from build123d import *

# Parameters (mm, degrees)
PAD_DEPTH    = 3
POCKET_DEPTH = 5
CHAMFER_SIZE = 1
FILLET_R     = 1


with BuildPart() as part:
    # Sketch → Pad (new body)
    with BuildSketch(Plane.XY):
        with BuildLine():
            Line((0, 15), (0, 0))
            Line((0, 0), (15, 0))
            Line((15, 0), (30, 3))
            ThreePointArc((30, -1.343534), (32.171767, 0.828233), (30, 3))
            Line((30, -1.343534), (24.21767, -2.5))
            ThreePointArc((24.21767, -2.5), (35.775711, -2.511474), (30, 7.5))
            ThreePointArc((30, 7.5), (35.775711, 17.511474), (24.21767, 17.5))
            Line((24.21767, 17.5), (30, 16.343534))
            ThreePointArc((30, 12), (32.171767, 14.171767), (30, 16.343534))
            Line((15, 15), (30, 12))
            Line((0, 15), (15, 15))
        make_face()
    extrude(amount=PAD_DEPTH)

    # Sketch001 (on Face13 of Pad) → Pocket (cut)
    with BuildSketch(Plane.XY.offset(3)):
        with BuildLine():
            ThreePointArc((7, 12.5), (6, 13.5), (5, 12.5))
            Line((5, 12.5), (5, 2.5))
            ThreePointArc((5, 2.5), (6, 1.5), (7, 2.5))
            Line((7, 12.5), (7, 2.5))
        make_face()
        with BuildLine():
            ThreePointArc((12, 12.5), (11, 13.5), (10, 12.5))
            Line((10, 12.5), (10, 2.5))
            ThreePointArc((10, 2.5), (11, 1.5), (12, 2.5))
            Line((12, 12.5), (12, 2.5))
        make_face()
    extrude(amount=-POCKET_DEPTH, mode=Mode.SUBTRACT)

    # Chamfer
    chamfer_edges = [part.edges().sort_by_distance(p)[0] for p in [
        (7, 7.5, 3),
        (10, 7.5, 3),
        (7, 7.5, 0),
        (10, 7.5, 0),
        (24.21767, 17.5, 1.5),
        (24.21767, -2.5, 1.5),
    ]]
    chamfer(chamfer_edges, length=CHAMFER_SIZE)

    # Fillet
    fillet_edges = [part.edges().sort_by_distance(p)[0] for p in [
        (0, 15, 1.5),
        (0, 0, 1.5),
    ]]
    fillet(fillet_edges, radius=FILLET_R)


solid = part.part
Can you work these out from the model? Positions are in its coordinate system, mm. A direction names the side the tool comes from. Give positions to 0.01 mm unless a question says otherwise; leave off trailing zeros. Loops run counter-clockwise (first coordinate to the right, second up) from the corner with the lowest first, then second, coordinate; pieces in that order, holes last. Notation, with made-up numbers: (-26.5, 12.5) -> (26.5, 12.5) arc R8 cw to (26.5, 27.5) -> close; hole circle Ø4 at (48, 45). An arc over 180 degrees is marked (long way). Write item = value, one per line.
1) For faces 1 (the flat face through (24.986, -2.823, 1.479)), 2 (the flat face through (8, 0, 1)), 3 (the conical face through (6, 1.2, 0.7)), 4 (the cylindrical face through (11, 1.5, 1.5)), which set-ups out of +Z, -Z, +X, -X, +Y, -Y let a thin tool reach every point of the face, with its end or its side?
Check result:
face_1 = +Z, -Z, -X
face_2 = +Z, -Z, -X, -Y
face_3 = -Z
face_4 = +Z, -Z
2) Will these pins go through, and if not, where does the flat tip stop? pin 1 (10 mm diameter, centred on x = 7, y = 14, fed in from -Z); pin 2 (1 mm diameter, centred on x = 22.5, z = 0.5, fed in from +Y); pin 3 (1.5 mm diameter, centred on x = 8, z = 1, fed in from +Y).
Check result:
pin_1 = 0
pin_2 = 13.6
pin_3 = 15
3) Suppose I cut it at B-B on z = 1.5. Write out the boundary of the cut face in (x, y).
Check result:
outline = (0, 1) arc R1 ccw to (1, 0) -> (15, 0) -> (30, 3) arc R2.17 cw to (30, -1.34) -> (25.2, -2.3) -> (24.78, -3.33) arc R6.67 ccw (long way) to (30, 7.5) arc R6.67 ccw (long way) to (24.78, 18.33) -> (25.2, 17.3) -> (30, 16.34) arc R2.17 cw to (30, 12) -> (15, 15) -> (1, 15) arc R1 ccw to (0, 14) -> close; hole (5, 2.5) arc R1 ccw to (7, 2.5) -> (7, 12.5) arc R1 ccw to (5, 12.5) -> close; hole (10, 2.5) arc R1 ccw to (12, 2.5) -> (12, 12.5) arc R1 ccw to (10, 12.5) -> close
4) Thinking about a two-plate mould opening in Y: for faces 5 (the cylindrical face through (32.17, 0.78, 1.48)), 6 (the cylindrical face through (35.925, -2.238, 1.479)), 7 (the flat face through (8, 15, 1)), 8 (the cylindrical face through (0.285, 0.301, 1.521)), which applies, released by +Y, released by -Y, zero draft, split by the parting line, or undercut?
Check result:
face_5 = undercut
face_6 = undercut
face_7 = released by +Y
face_8 = released by -Y
5) Suppose I cut it at C-C on x = 17.5. Write out the boundary of the cut face in (y, z).
Check result:
outline = (0.5, 0) -> (14.5, 0) -> (14.5, 3) -> (0.5, 3) -> close
6) Suppose I cut it at A-A on x = 11. Write out the boundary of the cut face in (y, z), then the cut area to 3 significant figures.
Check result:
outline = (0, 0) -> (0.5, 0) -> (1.5, 1) -> (1.5, 2) -> (0.5, 3) -> (0, 3) -> close; (13.5, 1) -> (14.5, 0) -> (15, 0) -> (15, 3) -> (14.5, 3) -> (13.5, 2) -> close
area = 7.00 mm2
7) I need wall thicknesses on L1, parallel to Y at x = 12, z = 0.2; L2, parallel to Y at x = 29.5, z = 1.7; L3, parallel to X at y = 6.5, z = 1.25. Which ranges of each line are inside material? Lowest first, please. Write a range as from..to.
Check result:
L1 = 0..1, 14..15
L2 = -5.82..-1.44, 2.9..12.1, 16.44..20.82
L3 = 0..5, 7..10, 12..33.51
8) Suppose I cut it at D-D on y = 19. Write out the boundary of the cut face in (x, z), then the cut area to 3 significant figures.
Check result:
outline = (25.4, 0) -> (34.6, 0) -> (34.6, 3) -> (25.4, 3) -> close
area = 27.6 mm2
